Could you check a few things on this model? Use its own coordinates, in mm. A direction names the side the tool comes from. Coordinates: 2 decimals unless noted, no trailing zeros. Write each loop counter-clockwise with the first axis right and the second up, starting at its lowest first coordinate (ties: lowest second). Pieces come first, ordered by that corner, then holes.
```python
from build123d import *

# Parameters (mm, degrees)
F0_R     = 15
F1_DEPTH = 33


with BuildPart() as f1:
    # F0 (on Top) → F1 (new body)
    with BuildSketch(Plane.XY):
        with BuildLine():
            ThreePointArc((-15.6397230178, 31.6627646983), (-9.8017078888, 1.6627646983), (-15.6397230178, -28.3372353017))
            ThreePointArc((-15.6397230178, -28.3372353017), (14.3602769822, -58.3372353017), (44.3602769822, -28.3372353017))
            ThreePointArc((44.3602769822, -28.3372353017), (38.5222618531, 1.6627646983), (44.3602769822, 31.6627646983))
            ThreePointArc((44.3602769822, 31.6627646983), (14.3602769822, 61.6627646983), (-15.6397230178, 31.6627646983))
        make_face()
        Polygon((-0.8574276546, -28.3372353017), (7.8028263832, -13.3372353017), (14.3602769822, -13.3372353017), (25.1233344589, -13.3372353017), (33.7835884968, -28.3372353017), (25.1233344589, -43.3372353017), (7.8028263832, -43.3372353017), align=None, mode=Mode.SUBTRACT)
        with Locations((14.3602769822, 31.6627646983)):
            Circle(F0_R, mode=Mode.SUBTRACT)
    extrude(amount=F1_DEPTH)


solid = f1.part
```
1. On a 3-axis mill with a long thin cutter (end or side, diameter ignored), from which of +Z, -Z, +X, -X, +Y, -Y can I reach the whole of each face in a straight line? I mean faces 4 (the face through (38.523, 1.232, 16.269)), 5 (the face through (3.53, -35.94, 16.27)). Say none if no direction works.
Verdict:
face 4: +Z, -Z, +X
face 5: +Z, -Z
2. If we mould it in two halves opening along X, with no side actions, what happens to faces 1 (the face through (14, 3, 33)), 2 (the face through (3.305, 41.8, 16.269)), 3 (the face through (15.02, 61.656, 16.269))? For each: pulls with the +X half, pulls with the -X half, needs draft (parallel to the pull), parting line crosses it, or undercut.
Verdict:
face 1: needs draft
face 2: undercut
face 3: parting line crosses it
3. I want a section at A-A on z = 25. Please give me the cut outline in (x, y), plus the area to 3 significant figures.
Verdict:
outline: (-15.64, -28.34) arc R30 ccw to (44.36, -28.34) arc R80 cw to (44.36, 31.66) arc R30 ccw to (-15.64, 31.66) arc R80 cw to start; hole (-0.86, -28.34) - (7.8, -43.34) - (25.12, -43.34) - (33.78, -28.34) - (25.12, -13.34) - (7.8, -13.34) - close; hole circle Ø30 at (14.36, 31.66)
area: 4,470 mm2
4. I want a section at C-C on y = 35. Please give me the cut outline in (x, z).
Verdict:
outline: (-15.45, 0) - (-0.26, 0) - (-0.26, 33) - (-15.45, 33) - close; (28.98, 0) - (44.17, 0) - (44.17, 33) - (28.98, 33) - close
5. For pin 1 (8 mm diameter, centred on x = 26.5, z = 26, fed in from +Y); pin 2 (8 mm diameter, centred on y = -7, z = 19, fed in from +X); pin 3 (12 mm diameter, centred on x = 18.5, z = 18.5, fed in from -Y), each with a flat end and sliding along its axis, tell me the tip position at first contact or that it passes through.
Verdict:
pin 1: stops at y = 60.54
pin 2: stops at x = 39.53
pin 3: stops at y = -58.34
6. Please list where these lines run through material, in increasing order: line 1 along Y through (x, z) = (9.5, 16); line 2 along Y through (x, z) = (27.5, 3.5); line 3 along X through (y, z) = (-35, 28).
Verdict:
line 1: y = -57.94 to -43.34, -13.34 to 17.47, 45.85 to 61.27
line 2: y = -55.31 to -39.22, -17.45 to 24.43, 38.9 to 58.63
line 3: x = -14.89 to 2.99, 29.94 to 43.61
7. I want a section at B-B on x = 13. Please give me the cut outline in (y, z), plus the area to 3 significant figures.
Verdict:
outline: (-58.31, 0) - (-43.34, 0) - (-43.34, 33) - (-58.31, 33) - close; (-13.34, 0) - (16.72, 0) - (16.72, 33) - (-13.34, 33) - close; (46.6, 0) - (61.63, 0) - (61.63, 33) - (46.6, 33) - close
area: 1,980 mm2
8. I want a section at D-D on x = 0.5. Please give me the cut outline in (y, z), plus the area to 3 significant figures.
Verdict:
outline: (-54.94, 0) - (-30.69, 0) - (-30.69, 33) - (-54.94, 33) - close; (-25.99, 0) - (25.93, 0) - (25.93, 33) - (-25.99, 33) - close; (37.4, 0) - (58.27, 0) - (58.27, 33) - (37.4, 33) - close
area: 3,200 mm2
